Verification items for this drawing (mm, ordinates from the low corner). A direction names the side the tool comes from. Coordinates: 2 decimals unless noted, no trailing zeros. Write each loop counter-clockwise with the first axis right and the second up, starting at its lowest first coordinate (ties: lowest second). Pieces come first, ordered by that corner, then holes. Notation, with made-up numbers: (-23, 47) -> (-13, 47) arc R12 ccw to (-13, 69) -> close; hole circle Ø5 at (78, -16). An arc over 180 degrees is marked (long way). Answer as CSV lines item,"result".
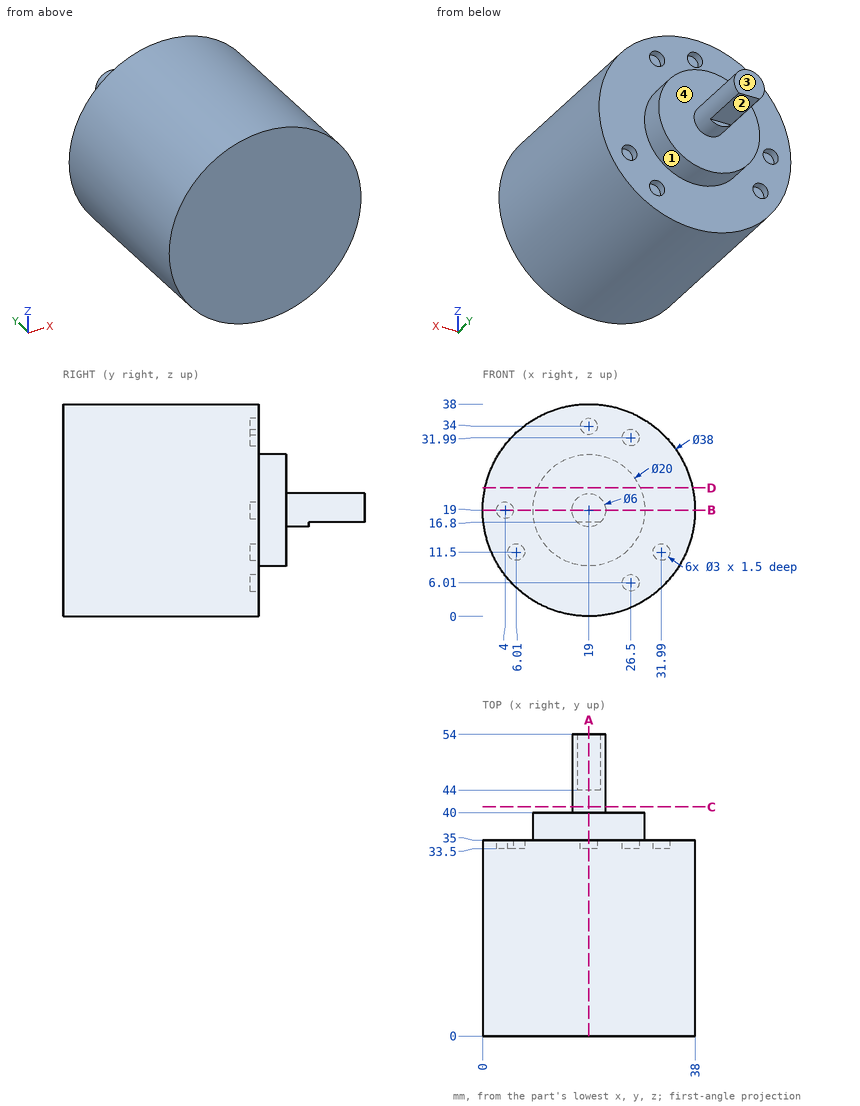
Item 1: Cross-section at C-C, the plane y = 41. Record the cut outline in (x, z), plus the area to 3 significant figures.
Responses:
outline,"circle Ø6 at (19, 19)"
area,"28.3 mm2"
Item 2: Depth check by flat-ended pin: pin 1 Ø2.5 at (x, z) = (5.5, 11) entering from +Y; pin 2 Ø6 at (x, y) = (19, 14.5) entering from +Z; pin 3 Ø5 at (y, z) = (30, 10.5) entering from +X. Enter the tip coordinate at first touch or a pass-through.
Responses:
pin 1,"stops at y = 35"
pin 2,"stops at z = 38"
pin 3,"stops at x = 37.03"
Item 3: Cross-section at B-B, the plane z = 19. Record the cut outline in (x, y), plus the area to 3 significant figures.
Responses:
outline,"(0, 0) -> (38, 0) -> (38, 35) -> (29, 35) -> (29, 40) -> (22, 40) -> (22, 54) -> (16, 54) -> (16, 40) -> (9, 40) -> (9, 35) -> (5.5, 35) -> (5.5, 33.5) -> (2.5, 33.5) -> (2.5, 35) -> (0, 35) -> close"
area,"1,510 mm2"
Item 4: Release check for a two-part mould opening along X. For the marked faces 1 and 2 record: +X half, -X half, draft (parallel to the pull), parting line (faces both ways), or undercut.
Responses:
face 1,"parting line"
face 2,"draft"
Item 5: Cross-section at D-D, the plane z = 23. Record the cut outline in (x, y) (1 decimal), plus the area to 3 significant figures.
Responses:
outline,"(0.4, 0) -> (37.6, 0) -> (37.6, 35) -> (28.2, 35) -> (28.2, 40) -> (9.8, 40) -> (9.8, 35) -> (0.4, 35) -> close"
area,"1,390 mm2"
Item 6: Cross-section at A-A, the plane x = 19. Record the cut outline in (y, z), plus the area to 3 significant figures.
Responses:
outline,"(0, 0) -> (35, 0) -> (35, 9) -> (40, 9) -> (40, 16) -> (44, 16) -> (44, 16.8) -> (54, 16.8) -> (54, 22) -> (40, 22) -> (40, 29) -> (35, 29) -> (35, 32.5) -> (33.5, 32.5) -> (33.5, 35.5) -> (35, 35.5) -> (35, 38) -> (0, 38) -> close"
area,"1,500 mm2"
Item 7: Set-up check for the marked faces 3 and 4: record each of +Z, -Z, +X, -X, +Y, -Y from which the full face is reachable in a straight line by a thin tool's end or side.
Responses:
face 3,"+Z, -Z, +X, -X, +Y"
face 4,"+Y"
Item 8: Thickness scan on probe 1 along Z at (x, y) = (19, 34.65); probe 2 along Z at (x, y) = (26.5, 34.7); probe 3 along Y at (x, z) = (22, 13). Record the ranges inside material, lowest first.
Responses:
probe 1,"z = 0 to 32.5, 35.5 to 38"
probe 2,"z = 1.54 to 4.51, 7.51 to 30.49, 33.49 to 36.46"
probe 3,"y = 0 to 40"
